from build123d import *

# Parameters (mm, degrees)
EXTRUDE_START       = 6
EXTRUDE_1_DEPTH     = 30
SKETCH_4_R          = 32
SKETCH_4_R_2        = 2.5
CUT_EXTRUDE_1_DEPTH = 2
CUT_EXTRUDE_1_DRAFT = -60
SKETCH_5_R          = 32
SKETCH_5_R_2        = 2.5
CUT_EXTRUDE_2_DEPTH = 2
CUT_EXTRUDE_2_DRAFT = -60
SKETCH_6_W          = 6
SKETCH_6_H          = 2
EXTRUDE1_START      = -15
SKETCH1_R           = 2
EXTRUDE1_DEPTH      = 15


with BuildPart() as part:
    # 草图3 → 凸台-拉伸1 (new body)
    with BuildSketch(Plane(origin=(0, 0, 0), x_dir=(0, 0, -1), z_dir=(1, 0, 0)).offset(EXTRUDE_START)):
        Polygon((2.5, 1.443375673), (0, 2.886751346), (-2.5, 1.443375673), (-2.5, -1.443375673), (0, -2.886751346), (2.5, -1.443375673), align=None)
    extrude(amount=EXTRUDE_1_DEPTH)


with BuildPart() as cut_extrude_1_tool:
    # 草图4 → 切除-拉伸1 (with draft: the straight prism first)
    with BuildSketch(Plane.ZY.offset(-6)):
        Circle(SKETCH_4_R)
        Circle(SKETCH_4_R_2, mode=Mode.SUBTRACT)
    extrude(amount=-CUT_EXTRUDE_1_DEPTH)
    # 切除-拉伸1: the draft: its side faces are tilted about the plane it starts from
    cut_extrude_1_sides = [cut_extrude_1_tool.faces().sort_by_distance(p)[0] for p in [
        (7, 0, -32),
        (7, 0, -2.5),
    ]]
    draft(cut_extrude_1_sides, Plane.ZY.offset(-6), CUT_EXTRUDE_1_DRAFT)


with BuildPart() as part_1:
    add(part.part)

    # 切除-拉伸1: cut by cut_extrude_1_tool
    add(cut_extrude_1_tool.part, mode=Mode.SUBTRACT)


with BuildPart() as cut_extrude_2_tool:
    # 草图5 → 切除-拉伸2 (with draft: the straight prism first)
    with BuildSketch(Plane(origin=(36, 0, 0), x_dir=(0, 0, -1), z_dir=(1, 0, 0))):
        Circle(SKETCH_5_R)
        Circle(SKETCH_5_R_2, mode=Mode.SUBTRACT)
    extrude(amount=-CUT_EXTRUDE_2_DEPTH)
    # 切除-拉伸2: the draft: its side faces are tilted about the plane it starts from
    cut_extrude_2_sides = [cut_extrude_2_tool.faces().sort_by_distance(p)[0] for p in [
        (35, 0, 32),
        (35, 0, 2.5),
    ]]
    draft(cut_extrude_2_sides, Plane(origin=(36, 0, 0), x_dir=(0, 0, -1), z_dir=(1, 0, 0)), CUT_EXTRUDE_2_DRAFT)


with BuildPart() as part_2:
    add(part_1.part)

    # 切除-拉伸2: cut by cut_extrude_2_tool
    add(cut_extrude_2_tool.part, mode=Mode.SUBTRACT)

    # 草图6 → 旋转1 (revolve)
    with BuildSketch(Plane.XY, mode=Mode.PRIVATE) as revolve_1_sk:
        with Locations((3, 1)):
            Rectangle(SKETCH_6_W, SKETCH_6_H)
    revolve(revolve_1_sk.sketch.rotate(Axis((0, 0, 0), (1, 0, 0)), 90), axis=Axis((0, 0, 0), (1, 0, 0)))

    # Sketch1 → Extrude1 (cut)
    with BuildSketch(Plane(origin=(36, 0, 0), x_dir=(0, 0, -1), z_dir=(1, 0, 0)).offset(EXTRUDE1_START)):
        with Locations(Location((0, 0, 0), (0, 0, 180))):
            Circle(SKETCH1_R)
    extrude(amount=EXTRUDE1_DEPTH, mode=Mode.SUBTRACT)


solid = part_2.part
Work out the finished part from the listing and answer in its coordinate system (mm). A direction names the side the tool comes from. Round coordinates to 2 decimals unless told otherwise and drop trailing zeros. Loops run counter-clockwise (first coordinate to the right, second up) from the corner with the lowest first, then second, coordinate; pieces in that order, holes last. Notation, with made-up numbers: (-12, 41.25) - (46, 41.25) arc R17 ccw to (46, 54.25) - close; hole circle Ø6 at (30, 33.5). An arc over 180 degrees is marked (long way). One line per item, written item: value.
Q1. Find section C-C on x = 4.5. Give the vertices of the cut face in (y, z).
Check values:
outline: circle Ø4 at (0, 0)
Q2. Straight lines are drawn through the part: probe 1 along X at (y, z) = (0.45, 0.25); probe 2 along X at (y, z) = (2, -0.75); probe 3 along Z at (x, y) = (11, -2.05). For each, find the intervals that lie inside material, in ascending order.
Check values:
probe 1: 0 to 21
probe 2: 6 to 36
probe 3: -1.45 to 1.45
Q3. Find section A-A on x = 28. Give the vertices of the cut face in (y, z).
Check values:
outline: (-2.89, 0) - (-1.44, -2.5) - (1.44, -2.5) - (2.89, 0) - (1.44, 2.5) - (-1.44, 2.5) - close; hole circle Ø4 at (0, 0)
Q4. This flat-tipped pin is pushed along its axis until it touches: pin 1 Ø2 at (y, z) = (0.5, -0.5) entering from +X. Where does it stop, or does it pass through?
Check values:
pin 1: x = 21
Q5. For faces 1 (the flat face through (20.79, 2.175, 1.233)), 2 (the flat face through (21, 0, 0)), 3 (the flat face through (6, 2, 1)), determine the directions among +Z, -Z, +X, -X, +Y, -Y from which every point of the face is accessible in a straight line to the end or side of a thin tool.
Check values:
face 1: +Z, +X, -X, +Y
face 2: +X
face 3: -X
Q6. The mould has two halves that part along Y. Classify faces 4 (the conical face through (35.922, 1.323, 2.279)), 5 (the cylindrical face through (3, 2, 0)), 6 (the cylindrical face through (28, 2, 0)): +Y half, -Y half, draft (parallel to the pull), parting line (faces both ways), or undercut.
Check values:
face 4: +Y half
face 5: parting line
face 6: undercut
Q7. Find section B-B on x = 12. Give the vertices of the cut face in (y, z), and give its area (3 significant figures).
Check values:
outline: (-2.89, 0) - (-1.44, -2.5) - (1.44, -2.5) - (2.89, 0) - (1.44, 2.5) - (-1.44, 2.5) - close
area: 21.7 mm2
